Design review of the part built by this model. Coordinates are the model's own, in mm. A direction names the side the tool comes from. Give positions to 0.01 mm unless a question says otherwise; leave off trailing zeros. Loops run counter-clockwise (first coordinate to the right, second up) from the corner with the lowest first, then second, coordinate; pieces in that order, holes last. Notation, with made-up numbers: M 77.25,-34 L 113.25,-34 A13 cw 113.25,-17 Z; hole C 65.25,53.25 d4. An arc over 180 degrees is marked long. Use one line per item in the form item = value. Start each with the question number.
from build123d import *

# Parameters (mm, degrees)
F0_R     = 2.794
F1_DEPTH = 1.27
F3_DEPTH = 1.778
F4_R     = 1.4097
F5_DEPTH = 12.7
F6_R     = 1.27


with BuildPart() as f1:
    # F0 (on Right) → F1 (new body)
    with BuildSketch(Plane.YZ):
        Circle(F0_R)
    extrude(amount=F1_DEPTH)

    # F2 (on face) → F3 (join)
    with BuildSketch(Plane.YZ.offset(1.27)):
        Polygon((-1.623683, -1.933988), (0.863042, -2.373145), (2.486725, -0.439157), (1.623683, 1.933988), (-0.863042, 2.373145), (-2.486725, 0.439157), align=None)
        Polygon((2.080505, -0.384262), (0.707472, -1.993901), (-1.373033, -1.609639), (-2.080505, 0.384262), (-0.707472, 1.993901), (1.373033, 1.609639), align=None, mode=Mode.SUBTRACT)
    extrude(amount=F3_DEPTH)

    # F4 (on face) → F5 (join)
    with BuildSketch(Plane(origin=(0, 0, 0), x_dir=(0, -1, 0), z_dir=(-1, 0, 0))):
        Circle(F4_R)
    extrude(amount=F5_DEPTH)

    # F6
    f6_edges = [f1.edges().sort_by_distance(p)[0] for p in [
        (-12.7, 1.4097, 0),
    ]]
    fillet(f6_edges, radius=F6_R)


solid = f1.part
Q1. Wall thickness on probe 1 along X at (y, z) = (1.7, 2); probe 2 along X at (y, z) = (-1.15, 1.9); probe 3 along Y at (x, z) = (-7, 0.3): over which ranges is each line inside the solid? List them lowest first.
Q2. For faces 5 (the cylindrical face through (-5.635, 0.306, -1.376)), 6 (the flat face through (2.147, 1.664, -1.42)), 7 (the flat face through (2.15, 2.06, 0.73)), 8 (the flat face through (2.15, -1.72, -0.63)), 9 (the flat face through (2.15, -0.4, -2.15)), list the 3-axis set-ups (+Z, -Z, +X, -X, +Y, -Y) from which the entire face can be reached by the end or side of a thin tool; tool diameter is ignored.
Q3. Take a section at B-B on x = -0.75. Give the boundary of the cut face in (y, z).
Q4. The part is to be moulded in two halves that separate along Z. For faces 1 (the flat face through (0, 1.2, -1.2)), 2 (the flat face through (2.15, -2.06, -0.73)), 3 (the flat face through (2.147, -0.318, -1.804)), 4 (the flat face through (2.15, 0.4, 2.15)), say which applies: pulls with the +Z half, pulls with the -Z half, needs draft (parallel to the pull), parting line crosses it, or undercut.
Q5. Clearance check with flat-ended pins moving along their axes: pin 1 Ø1.5 at (x, z) = (-11, 0.5) entering from -Y; pin 2 Ø1.2 at (y, z) = (-0.5, -0.5) entering from +X; pin 3 Ø1.5 at (x, y) = (-6.5, -0.5) entering from -Z. State where each tip first meets the part, or that it passes through.
Q6. Take a section at A-A on x = 1.5. Give the boundary of the cut face in (y, z), plus the area to 3 significant figures.
Response values:
q1.probe_1 = 0 to 1.27
q1.probe_2 = 0 to 3.05
q1.probe_3 = -1.38 to 1.38
q2.face_5 = -X
q2.face_6 = -Z, +X, +Y
q2.face_7 = +Z, +X, +Y
q2.face_8 = +X
q2.face_9 = -Z, +X, -Y
q3.outline = C 0,0 d2.82
q4.face_1 = needs draft
q4.face_2 = pulls with the -Z half
q4.face_3 = undercut
q4.face_4 = pulls with the +Z half
q5.pin_1 = -1.41
q5.pin_2 = 1.27
q5.pin_3 = -1.41
q6.outline = M -2.49,0.44 L -1.62,-1.93 L 0.86,-2.37 L 2.49,-0.44 L 1.62,1.93 L -0.86,2.37 Z; hole M -2.08,0.38 L -1.37,-1.61 L 0.71,-1.99 L 2.08,-0.38 L 1.37,1.61 L -0.71,1.99 Z
q6.area = 4.94 mm^2
